```python
from build123d import *

# Parameters (mm, degrees)
SKETCH1_W           = 92.2
SKETCH1_H           = 81.1
BOSS_EXTRUDE1_DEPTH = 4.2
CUT_EXTRUDE1_DEPTH  = 4.6
CUT_EXTRUDE2_DEPTH  = 9.4
CUT_EXTRUDE3_DEPTH  = 9.4
SKETCH5_R           = 2.35
SKETCH5_R_2         = 1.9
CUT_EXTRUDE4_DEPTH  = 1.5
SKETCH6_W           = 1.4
SKETCH6_H           = 81.1
CUT_EXTRUDE5_DEPTH  = 9.4


with BuildPart() as part:
    # Sketch1 → Boss-Extrude1 (new body, symmetric)
    with BuildSketch(Plane(origin=(0, 0, 0), x_dir=(1, 0, 0), z_dir=(0, 1, 0))):
        Rectangle(SKETCH1_W, SKETCH1_H)
    extrude(amount=BOSS_EXTRUDE1_DEPTH, both=True)

    # Sketch2 → Cut-Extrude1 (cut)
    with BuildSketch(Plane.XZ.offset(4.2)):
        with BuildLine():
            Line((38.85, 40.55), (34.85, 40.55))
            Line((34.85, 40.55), (32.35, 40.55))
            ThreePointArc((32.35, 40.55), (34.117766953, 39.817766953), (34.85, 38.05))
            Line((34.85, 38.05), (34.85, 36.55))
            Line((34.85, 36.55), (38.85, 36.55))
            Line((38.85, 36.55), (38.85, 40.55))
        make_face()
        with BuildLine():
            Line((22.85, 36.55), (26.85, 36.55))
            Line((26.85, 36.55), (26.85, 38.05))
            ThreePointArc((26.85, 38.05), (27.582233047, 39.817766953), (29.35, 40.55))
            Line((29.35, 40.55), (26.85, 40.55))
            Line((26.85, 40.55), (22.85, 40.55))
            Line((22.85, 40.55), (22.85, 36.55))
        make_face()
        with BuildLine():
            Line((22.85, -36.55), (22.85, -40.55))
            Line((22.85, -40.55), (29.35, -40.55))
            ThreePointArc((29.35, -40.55), (27.582233047, -39.817766953), (26.85, -38.05))
            Line((26.85, -38.05), (26.85, -36.55))
            Line((26.85, -36.55), (22.85, -36.55))
        make_face()
        with BuildLine():
            Line((34.85, -36.55), (34.85, -38.05))
            ThreePointArc((34.85, -38.05), (34.117766953, -39.817766953), (32.35, -40.55))
            Line((32.35, -40.55), (38.85, -40.55))
            Line((38.85, -40.55), (38.85, -36.55))
            Line((38.85, -36.55), (34.85, -36.55))
        make_face()
    extrude(amount=-CUT_EXTRUDE1_DEPTH, mode=Mode.SUBTRACT)

    # Sketch3 → Cut-Extrude2 (cut, through all)
    with BuildSketch(Plane.XZ.offset(4.2)):
        with BuildLine():
            Line((45, 40.55), (46.1, 40.55))
            Line((46.1, 40.55), (46.1, 34.4))
            Line((46.1, 34.4), (45.5, 34.4))
            ThreePointArc((45.5, 34.4), (45.146446609, 34.546446609), (45, 34.9))
            Line((45, 34.9), (45, 40.55))
        make_face()
        with BuildLine():
            Line((46.1, -34.4), (46.1, -40.55))
            Line((46.1, -40.55), (45, -40.55))
            Line((45, -40.55), (45, -34.9))
            ThreePointArc((45, -34.9), (45.146446609, -34.546446609), (45.5, -34.4))
            Line((45.5, -34.4), (46.1, -34.4))
        make_face()
        with BuildLine():
            Line((-46.1, -37.767949192), (-46.1, -40.55))
            Line((-46.1, -40.55), (-45.397795547, -40.55))
            ThreePointArc((-45.397795547, -40.55), (-45.160817466, -39.010539992), (-46.1, -37.767949192))
        make_face()
        with BuildLine():
            Line((-46.1, -14.767949192), (-46.1, -18.232050808))
            ThreePointArc((-46.1, -18.232050808), (-45.1, -16.5), (-46.1, -14.767949192))
        make_face()
        with BuildLine():
            Line((-46.1, 18.232050808), (-46.1, 14.767949192))
            ThreePointArc((-46.1, 14.767949192), (-45.1, 16.5), (-46.1, 18.232050808))
        make_face()
        with BuildLine():
            Line((-45.397795547, 40.55), (-46.1, 40.55))
            Line((-46.1, 40.55), (-46.1, 37.767949192))
            ThreePointArc((-46.1, 37.767949192), (-45.160817466, 39.010539992), (-45.397795547, 40.55))
        make_face()
    extrude(amount=-CUT_EXTRUDE2_DEPTH, mode=Mode.SUBTRACT)

    # Sketch4 → Cut-Extrude3 (cut, through all)
    with BuildSketch(Plane.XZ.offset(4.2)):
        Polygon((-38.632, 11.8872), (-38.632, 12.2428), (-38.632, 14.2875), (-40.537, 14.2875), (-46.125, 14.2875), (-46.125, 13.6525), (-46.125, -14.2875), (-40.537, -14.2875), (-38.632, -14.2875), (-38.632, -12.2428), (-38.632, -11.8872), align=None)
    extrude(amount=-CUT_EXTRUDE3_DEPTH, mode=Mode.SUBTRACT)

    # Sketch5 → Cut-Extrude4 (cut)
    with BuildSketch(Plane.XZ.offset(4.2)):
        with Locations((41.25, -25)):
            Circle(SKETCH5_R)
        with Locations((41.25, 25)):
            Circle(SKETCH5_R)
        with Locations((19.5, 0)):
            Circle(SKETCH5_R)
        with Locations((-1.3, 15)):
            Circle(SKETCH5_R_2)
        with Locations((-1.3, -15)):
            Circle(SKETCH5_R_2)
        with Locations((-22.1, 0)):
            Circle(SKETCH5_R)
        with Locations((-43.85, -25)):
            Circle(SKETCH5_R)
        with Locations((-43.85, 25)):
            Circle(SKETCH5_R)
    extrude(amount=-CUT_EXTRUDE4_DEPTH, mode=Mode.SUBTRACT)

    # Sketch6 → Cut-Extrude5 (cut, through all)
    with BuildSketch(Plane.XZ.offset(4.2)):
        with Locations((45.4, 0)):
            Rectangle(SKETCH6_W, SKETCH6_H)
    extrude(amount=-CUT_EXTRUDE5_DEPTH, mode=Mode.SUBTRACT)


solid = part.part
```
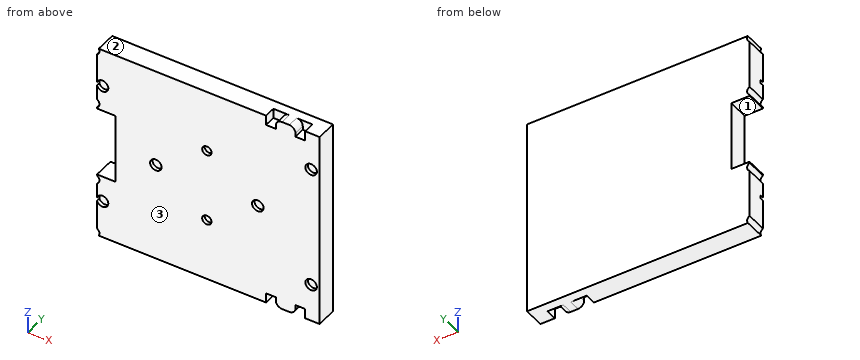
Geometry check sheet. Reference: the model listing, model coordinates, mm. Face numbers are marked on the shaded views. Coordinates: 2 decimals unless noted, no trailing zeros. Order: outer loops, then holes, each group sorted by start corner. A loop starts at its lowest first (then second) coordinate and runs counter-clockwise, first axis right, second up.
Item 1: Scan lines: line 1 along Z through (x, y) = (41.25, -3.45); line 2 along Z through (x, y) = (-43.85, -3.85); line 3 along Z through (x, y) = (-1.3, -3.1). Record each from-to range of solid material in increasing order.
Item 2: Section check D-D (z = -8). Enter the section's corners in (x, y), plus the area to 3 significant figures.
Item 3: Depth check by flat-ended pin: pin 1 (1.1 mm diameter, centred on x = -0.5, z = -16, fed in from -Y); pin 2 (2.5 mm diameter, centred on y = -1, z = -7, fed in from -X). Enter the tip coordinate at first touch or a pass-through.
Item 4: Section check B-B (x = 41.25). Enter the section's corners in (y, z), plus the area to 3 significant figures.
Item 5: Section check A-A (x = -43.85). Enter the section's corners in (y, z), plus the area to 3 significant figures.
Item 6: Section check C-C (y = 1.5). Enter the section's corners in (x, z), plus the area to 3 significant figures.
Item 7: Mould release check, pull along Z, two halves, no side actions. Record for the marked faces 1, 2 and 3: released by +Z, released by -Z, zero draft, split by the parting line, or undercut.
Check sheet entries:
1. line 1: z = -40.55 to -27.35, -22.65 to 22.65, 27.35 to 40.55
1. line 2: z = -40.55 to -27.35, -22.65 to -14.29, 14.29 to 22.65, 27.35 to 40.55
1. line 3: z = -40.55 to -16.9, -13.1 to 13.1, 16.9 to 40.55
2. outline: (-38.63, -4.2) - (44.7, -4.2) - (44.7, 4.2) - (-38.63, 4.2) - close
2. area: 700 mm2
3. pin 1: stops at y = -2.7
3. pin 2: stops at x = -38.63
4. outline: (-4.2, -40.55) - (4.2, -40.55) - (4.2, 40.55) - (-4.2, 40.55) - (-4.2, 27.35) - (-2.7, 27.35) - (-2.7, 22.65) - (-4.2, 22.65) - (-4.2, -22.65) - (-2.7, -22.65) - (-2.7, -27.35) - (-4.2, -27.35) - close
4. area: 667 mm2
5. outline: (-4.2, -40.55) - (4.2, -40.55) - (4.2, -14.29) - (-4.2, -14.29) - (-4.2, -22.65) - (-2.7, -22.65) - (-2.7, -27.35) - (-4.2, -27.35) - close; (-4.2, 14.29) - (4.2, 14.29) - (4.2, 40.55) - (-4.2, 40.55) - (-4.2, 27.35) - (-2.7, 27.35) - (-2.7, 22.65) - (-4.2, 22.65) - close
5. area: 427 mm2
6. outline: (-46.1, -37.77) arc R2 cw to (-45.4, -40.55) - (44.7, -40.55) - (44.7, 40.55) - (-45.4, 40.55) arc R2 cw to (-46.1, 37.77) - (-46.1, 18.23) arc R2 cw to (-46.1, 14.77) - (-46.1, 14.29) - (-38.63, 14.29) - (-38.63, -14.29) - (-46.1, -14.29) - (-46.1, -14.77) arc R2 cw to (-46.1, -18.23) - close
6. area: 7,140 mm2
7. face 1: undercut
7. face 2: released by +Z
7. face 3: zero draft
